from build123d import *

# Parameters (mm, degrees)
F1_DEPTH = 21.844
F2_R     = 30.1592813174
F3_DEPTH = 62.484
F4_R     = 19.5786544463
F5_DEPTH = 62.738
F7_DEPTH = 23.876
F8_R     = 7.0578530297
F9_DEPTH = 33.02


with BuildPart() as f1:
    # F0 (on Top) → F1 (new body)
    with BuildSketch(Plane.XY):
        with BuildLine():
            Line((-62.3466224072, 23.7019382979), (-61.5820136192, 23.6970914847))
            ThreePointArc((-61.5820136192, 23.6970914847), (-61.9642984681, 23.7025982274), (-62.3466224072, 23.7019382979))
        make_face()
        with BuildLine():
            Line((-41.3086953744, 23.5685800324), (-61.5820136192, 23.6970914847))
            Line((-61.5820136192, 23.6970914847), (-62.3466224072, 23.7019382979))
            ThreePointArc((-62.3466224072, 23.7019382979), (-85.8168487149, -0.1915085468), (-61.9636058746, -23.702593827))
            Line((-61.9636058746, -23.702593827), (-41.3055604078, -23.5710399543))
            ThreePointArc((-41.3055604078, -23.5710399543), (-52.7722777928, -0.0019924377), (-41.3086953744, 23.5685800324))
        make_face()
        with BuildLine():
            ThreePointArc((-4.0190974569, 23.3322033166), (-22.6226378881, 29.9591287907), (-41.3086953744, 23.5685800324))
            Line((-41.3086953744, 23.5685800324), (-4.0190974569, 23.3322033166))
        make_face()
        with BuildLine():
            Line((-4.0190974569, 23.3322033166), (-41.3086953744, 23.5685800324))
            ThreePointArc((-41.3086953744, 23.5685800324), (-52.7722777928, -0.0019924377), (-41.3055604078, -23.5710399543))
            Line((-41.3055604078, -23.5710399543), (-4.020837331, -23.3336046305))
            ThreePointArc((-4.020837331, -23.3336046305), (4.211331439, -12.9342741883), (7.1471835347, 0))
            ThreePointArc((7.1471835347, 0), (4.2118136579, 12.933266629), (-4.0190974569, 23.3322033166))
        make_face()
        with BuildLine():
            Line((43.5569020036, 23.0306216657), (-4.0190974569, 23.3322033166))
            ThreePointArc((-4.0190974569, 23.3322033166), (4.2118136579, 12.933266629), (7.1471835347, 0))
            ThreePointArc((7.1471835347, 0), (4.211331439, -12.9342741883), (-4.020837331, -23.3336046305))
            Line((-4.020837331, -23.3336046305), (43.5569020036, -23.0306216657))
            ThreePointArc((43.5569020036, -23.0306216657), (66.4419965279, 0), (43.5569020036, 23.0306216657))
        make_face()
        with BuildLine():
            Line((-4.020837331, -23.3336046305), (-41.3055604078, -23.5710399543))
            ThreePointArc((-41.3055604078, -23.5710399543), (-22.6217624778, -29.9591232288), (-4.020837331, -23.3336046305))
        make_face()
    extrude(amount=F1_DEPTH)

    # F2 (on Top) → F3 (join)
    with BuildSketch(Plane.XY):
        with Locations((-23.0502411723, 0)):
            Circle(F2_R)
    extrude(amount=F3_DEPTH)

    # F4 (on Top) → F5 (cut)
    with BuildSketch(Plane.XY):
        with Locations((-23.2811495662, 0)):
            Circle(F4_R)
    extrude(amount=F5_DEPTH, mode=Mode.SUBTRACT)

    # F6 (on Top) → F7 (cut)
    with BuildSketch(Plane.XY):
        with BuildLine():
            ThreePointArc((43.913397938, -7.536449256), (49.242472313, -5.329074375), (51.449847194, 0))
            ThreePointArc((51.449847194, 0), (49.2437269469, 5.3278194456), (43.9169469964, 7.5364484203))
            Line((43.9169469964, 7.5364484203), (43.913397938, -7.536449256))
        make_face()
        with BuildLine():
            Line((43.913397938, -7.536449256), (43.9169469964, 7.5364484203))
            ThreePointArc((43.9169469964, 7.5364484203), (36.3769488909, 0.0017745292), (43.913397938, -7.536449256))
        make_face()
        with BuildLine():
            ThreePointArc((43.913397938, -7.536449256), (36.3769488909, 0.0017745292), (43.9169469964, 7.5364484203))
            Line((43.9169469964, 7.5364484203), (20.3525681334, 7.5475453391))
            ThreePointArc((20.3525681334, 7.5475453391), (25.4034820207, 5.1836600837), (27.4600210391, 0))
            ThreePointArc((27.4600210391, 0), (25.2481571439, -5.3438018752), (19.9066354296, -7.5611665607))
            Line((19.9066354296, -7.5611665607), (43.913397938, -7.536449256))
        make_face()
        with BuildLine():
            ThreePointArc((27.4600210391, 0), (25.4034820207, 5.1836600837), (20.3525681334, 7.5475453391))
            ThreePointArc((20.3525681334, 7.5475453391), (12.3409711396, 0.2230703443), (19.9066354296, -7.5611665607))
            ThreePointArc((19.9066354296, -7.5611665607), (25.2481571439, -5.3438018752), (27.4600210391, 0))
        make_face()
    extrude(amount=F7_DEPTH, mode=Mode.SUBTRACT)

    # F8 (on Top) → F9 (cut)
    with BuildSketch(Plane.XY):
        with Locations((-66.9229701161, 0)):
            Circle(F8_R)
    extrude(amount=F9_DEPTH, mode=Mode.SUBTRACT)


solid = f1.part
Source: CAD feature listing. Evaluate the final solid. Frame: model axes, mm. A direction names the side the tool comes from. Coordinates: 2 decimals unless noted, no trailing zeros. Loops run counter-clockwise (first coordinate to the right, second up) from the corner with the lowest first, then second, coordinate; pieces in that order, holes last. Notation, with made-up numbers: (10.5, 87.5) -> (45.5, 87.5) arc R29 ccw to (45.5, 109.5) -> close; hole circle Ø8 at (74, 15.25). An arc over 180 degrees is marked (long way). Answer in a Markdown table with one row per item. Add a question column.
Q1. Section D-D on x = -1. Return the cut outline in (y, z), and give its area (3 significant figures).
Q2. Ray query, line 1 along X through (y, z) = (0, 17); line 2 along Y through (x, z) = (43.5, 17.5); line 3 along Y through (x, z) = (-23.5, 43.5). Return the intervals inside material, ascending.
Q3. Reachability of faces 1 (the face through (5.716, 9.059, 37.747)), 2 (the face through (-5.195, -7.499, 30.805)) from +Z, -Z, +X, -X, +Y, -Y: full face, straight path, thin tool, end or side. Return the list, or none.
Q4. Section A-A on z = 6. Return the cut outline in (x, y), and give its area (3 significant figures).
Q5. Contact query for flat-ended pins moving along their axis: pin 1 Ø6 at (x, z) = (-18.5, 34) entering from +Y; pin 2 Ø5 at (x, z) = (-67.5, 15) entering from -Y; pin 3 Ø6 at (x, z) = (-24, 40) entering from -Y; pin 4 Ø12 at (x, y) = (-16, -17.5) entering from +Z. Output: stop coordinate, or through.
Q6. Section C-C on y = -12.5. Return the cut outline in (x, z), and give its area (3 significant figures).
Q7. Section B-B on x = 16.5. Return the cut outline in (y, z).
Q8. Pull-direction query (Y, two-part tool) for faces 3 (the face through (66.436, -0.504, 10.769)), 4 (the face through (12.348, 0.392, 10.769)), 5 (the face through (6, 0, 0)); classes: pulls with the +Y half, pulls with the -Y half, needs draft (parallel to the pull), parting line crosses it, or undercut.
Computed values:
| question | item | result |
|---|---|---|
| 1 | outline | (-23.31, 0) -> (23.31, 0) -> (23.31, 21.84) -> (20.58, 21.84) -> (20.58, 62.48) -> (-20.58, 62.48) -> (-20.58, 21.84) -> (-23.31, 21.84) -> close |
| 1 | area | 2,690 mm^2 |
| 2 | line 1 | x = -85.82 to -73.98, -59.87 to -42.86, -3.7 to 12.34, 51.45 to 66.44 |
| 2 | line 2 | y = -23.03 to -7.54, 7.54 to 23.03 |
| 2 | line 3 | y = -30.16 to -19.58, 19.58 to 30.16 |
| 3 | face 1 | +Z |
| 3 | face 2 | +Z, -Z |
| 4 | outline | (-61.96, -23.7) -> (-41.86, -23.57) arc R30.16 ccw to (-3.94, -23.33) -> (43.56, -23.03) arc R23.03 ccw to (43.56, 23.03) -> (-3.94, 23.33) arc R30.16 ccw to (-41.86, 23.57) -> (-61.58, 23.7) arc R23.7 ccw (long way) to start; hole circle Ø14.12 at (-66.92, 0); hole circle Ø39.16 at (-23.28, 0); hole (19.91, -7.56) -> (43.91, -7.54) arc R7.54 ccw to (43.92, 7.54) -> (20.35, 7.55) arc R7.56 ccw (long way) to start |
| 4 | area | 5,090 mm^2 |
| 5 | pin 1 | stops at y = 30.12 |
| 5 | pin 2 | stops at y = -23.53 |
| 5 | pin 3 | stops at y = -30.16 |
| 5 | pin 4 | stops at z = 62.48 |
| 6 | outline | (-82.25, 0) -> (-38.35, 0) -> (-38.35, 62.48) -> (-50.5, 62.48) -> (-50.5, 21.84) -> (-82.25, 21.84) -> close; (-8.21, 0) -> (62.75, 0) -> (62.75, 21.84) -> (4.4, 21.84) -> (4.4, 62.48) -> (-8.21, 62.48) -> close |
| 6 | area | 3,520 mm^2 |
| 7 | outline | (-23.2, 0) -> (-6.75, 0) -> (-6.75, 21.84) -> (-23.2, 21.84) -> close; (6.75, 0) -> (23.2, 0) -> (23.2, 21.84) -> (6.75, 21.84) -> close |
| 8 | face 3 | parting line crosses it |
| 8 | face 4 | undercut |
| 8 | face 5 | needs draft |
